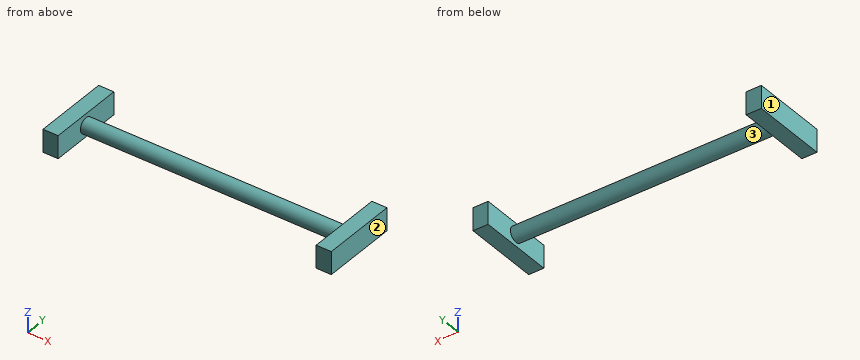
from build123d import *

# Parameters (mm, degrees)
F1_DEPTH = 38.1
F2_R     = 12.7
F3_DEPTH = 431.8
F4_W     = 127
F4_H     = 38.1
F5_DEPTH = 25.4


with BuildPart() as f1:
    # F0 (on Top) → F1 (new body)
    with BuildSketch(Plane.XY):
        Polygon((-46.300181, 91.77144), (-71.700181, 91.77144), (-71.700181, -35.22856), (-46.300181, -35.22856), (-46.300181, 15.57144), (-46.300181, 40.97144), align=None)
    extrude(amount=F1_DEPTH)

    # F2 (on face) → F3 (join)
    with BuildSketch(Plane.YZ.offset(-46.300181)):
        with Locations((28.27144, 19.05)):
            Circle(F2_R)
    extrude(amount=F3_DEPTH)

    # F4 (on face) → F5 (join)
    with BuildSketch(Plane.YZ.offset(385.499819)):
        with Locations((28.27144, 19.05)):
            Rectangle(F4_W, F4_H)
    extrude(amount=F5_DEPTH)


solid = f1.part
For this review, take the finished solid that the model builds, in its own axes (mm). Face numbers are marked on the shaded views. Round coordinates to 2 decimals unless told otherwise and drop trailing zeros. Write each loop counter-clockwise with the first axis right and the second up, starting at its lowest first coordinate (ties: lowest second). Pieces come first, ordered by that corner, then holes. Notation, with made-up numbers: (61.5, 79) -> (83.5, 79) arc R23 cw to (83.5, 111) -> close; hole circle Ø3 at (62.5, -35.75). An arc over 180 degrees is marked (long way). Put each result on its own line as item: value.
Q1. Consider section A-A on y = 57. State the section outline as (x, z) points.
Determined:
outline: (-71.7, 0) -> (-46.3, 0) -> (-46.3, 38.1) -> (-71.7, 38.1) -> close; (385.5, 0) -> (410.9, 0) -> (410.9, 38.1) -> (385.5, 38.1) -> close
Q2. Clearance check with flat-ended pins moving along their axes: pin 1 Ø8 at (x, z) = (-2, 31.5) entering from +Y; pin 2 Ø2 at (x, z) = (162, 12.5) entering from +Y; pin 3 Ø6 at (x, y) = (-10.5, 17.5) entering from -Z; pin 4 Ø10 at (x, y) = (228, 50.5) entering from -Z. State where each tip first meets the part, or that it passes through.
Determined:
pin 1: stops at y = 37.75
pin 2: stops at y = 39.69
pin 3: stops at z = 9.01
pin 4: passes through
Q3. Consider section D-D on y = 23.5. State the section outline as (x, z) points, and give its area (3 significant figures).
Determined:
outline: (-71.7, 0) -> (-46.3, 0) -> (-46.3, 7.28) -> (385.5, 7.28) -> (385.5, 0) -> (410.9, 0) -> (410.9, 38.1) -> (385.5, 38.1) -> (385.5, 30.82) -> (-46.3, 30.82) -> (-46.3, 38.1) -> (-71.7, 38.1) -> close
area: 12,100 mm^2
Q4. Consider section C-C on x = 31.5. State the section outline as (y, z) points.
Determined:
outline: circle Ø25.4 at (28.27, 19.05)
Q5. To check wall thickness, follow L1, parallel to X at y = 11, z = 35; L2, parallel to Y at x = 151, z = 18; L3, parallel to Y at x = 27.5, z = 30. State the ranges of each line that lie inside material, in increasing order. Write a range as [from, to].
Determined:
L1: x = [-71.7, -46.3], [385.5, 410.9]
L2: y = [15.61, 40.93]
L3: y = [21.84, 34.7]
Q6. The part is to be moulded in two halves that separate along X. For the marked faces 1, 2 and 3, say which applies: released by +X, released by -X, zero draft, split by the parting line, or undercut.
Determined:
face 1: released by -X
face 2: released by +X
face 3: undercut
Q7. Consider section B-B on z = 19.05. State the section outline as (x, y) points.
Determined:
outline: (-71.7, -35.23) -> (-46.3, -35.23) -> (-46.3, 15.57) -> (385.5, 15.57) -> (385.5, -35.23) -> (410.9, -35.23) -> (410.9, 91.77) -> (385.5, 91.77) -> (385.5, 40.97) -> (-46.3, 40.97) -> (-46.3, 91.77) -> (-71.7, 91.77) -> close
